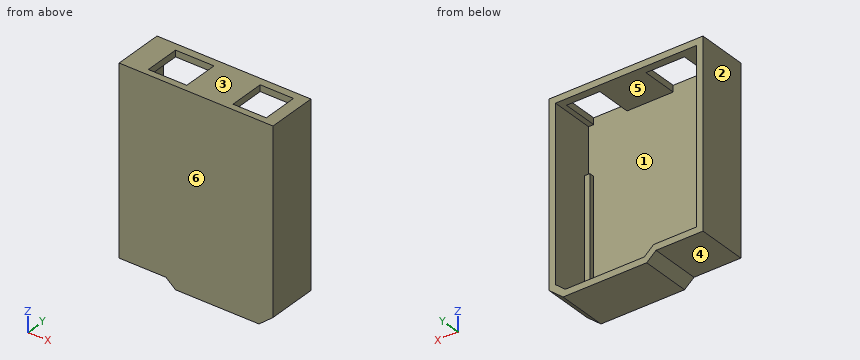
from build123d import *

# Parameters (mm, degrees)
BOSS_EXTRUDE1_DEPTH = 17
SHELL1_T            = 2.5
SKETCH2_W           = 15
SKETCH2_H           = 14
SKETCH2_W_2         = 13
CUT_EXTRUDE1_DEPTH  = 4
SKETCH3_W           = 2
SKETCH3_H           = 50
BOSS_EXTRUDE2_DEPTH = 2
SKETCH4_W           = 26.147040262
SKETCH4_H           = 2.874772828
BOSS_EXTRUDE3_DEPTH = 2


with BuildPart() as part:
    # Sketch1 → Boss-Extrude1 (new body)
    with BuildSketch(Plane(origin=(0, 0, 0), x_dir=(1, 0, 0), z_dir=(0, 1, 0))):
        Polygon((0, 0), (0, 67), (16.729272308, 67), (20.392796314, 70.176839536), (51.157808577, 70.176839536), (55, 67), (55, 0), align=None)
    extrude(amount=BOSS_EXTRUDE1_DEPTH)

    # Shell1
    shell1_openings = [part.faces().sort_by_distance(p)[0] for p in [
        (27.740476626, 17, -34.512318995),
    ]]
    offset(amount=SHELL1_T, openings=shell1_openings, kind=Kind.INTERSECTION)

    # Sketch2 → Cut-Extrude1 (cut)
    with BuildSketch(Plane(origin=(0, 0, 0), x_dir=(-1, 0, 0), z_dir=(0, 0, -1))):
        with Locations((-14.5, 7)):
            Rectangle(SKETCH2_W, SKETCH2_H)
        with Locations((-46.5, 7)):
            Rectangle(SKETCH2_W_2, SKETCH2_H)
    extrude(amount=-CUT_EXTRUDE1_DEPTH, mode=Mode.SUBTRACT)

    # Sketch3 → Boss-Extrude2 (add)
    with BuildSketch(Plane(origin=(0, 0, 0), x_dir=(1, 0, 0), z_dir=(0, 1, 0))):
        with Locations((1, 44.078139118)):
            Rectangle(SKETCH3_W, SKETCH3_H)
        with Locations((54, 44.078139118)):
            Rectangle(SKETCH3_W, SKETCH3_H)
    extrude(amount=BOSS_EXTRUDE2_DEPTH)

    # Sketch4 → Boss-Extrude3 (add)
    with BuildSketch(Plane(origin=(0, 0, 0), x_dir=(1, 0, 0), z_dir=(0, 1, 0))):
        with Locations((35.808300775, 68.739453122)):
            Rectangle(SKETCH4_W, SKETCH4_H)
    extrude(amount=BOSS_EXTRUDE3_DEPTH)


solid = part.part
Source: CAD feature listing. Evaluate the final solid. Frame: model axes, mm. Face numbers are marked on the shaded views. A direction names the side the tool comes from. Give positions to 0.01 mm unless a question says otherwise; leave off trailing zeros. Order: outer loops, then holes, each group sorted by start corner. A loop starts at its lowest first (then second) coordinate and runs counter-clockwise, first axis right, second up. Notation, with made-up numbers: (18.5, -33) -> (30.5, -33) arc R9 ccw to (30.5, -23) -> close; hole circle Ø8 at (-12.5, 62). An arc over 180 degrees is marked (long way). Use a Markdown table: item, result.
1) Contact query for flat-ended pins moving along their axis: P1, Ø1, axis at x = 4.5, z = -42.5, coming from the +Y side; P2, Ø1.6, axis at x = 53.5, z = -55.5, coming from the +Y side; P3, Ø8.5, axis at x = 11.5, y = 9.5, coming from the +Z side. Output: stop coordinate, or through.
Answer list:
| item | result |
|---|---|
| P1 | y = 0 |
| P2 | y = 2 |
| P3 | z = -67 |
2) Section query D-D, the plane x = 29. Return the cut outline in (y, z).
Answer list:
| item | result |
|---|---|
| outline | (-2.5, -72.68) -> (17, -72.68) -> (17, -70.18) -> (2, -70.18) -> (2, -67.3) -> (0, -67.3) -> (0, 0) -> (17, 0) -> (17, 2.5) -> (-2.5, 2.5) -> close |
3) Ray query, line 1 along Z through (x, y) = (28, 2.5); line 2 along X through (y, z) = (15.25, -38); line 3 along Z through (x, y) = (33, 0.5). Return the intervals inside material, ascending. Write a range as [from, to].
Answer list:
| item | result |
|---|---|
| line 1 | [-72.68, -70.18], [0, 2.5] |
| line 2 | [-2.5, 0], [55, 57.5] |
| line 3 | [-72.68, -67.3], [0, 2.5] |
4) Section query B-B, the plane y = 5.75. Return the cut outline in (x, z), then the cut area to 3 significant figures.
Answer list:
| item | result |
|---|---|
| outline | (-2.5, -69.5) -> (15.8, -69.5) -> (19.46, -72.68) -> (52.06, -72.68) -> (57.5, -68.18) -> (57.5, 2.5) -> (53, 2.5) -> (53, 0) -> (55, 0) -> (55, -67) -> (51.16, -70.18) -> (20.39, -70.18) -> (16.73, -67) -> (0, -67) -> (0, 0) -> (7, 0) -> (7, 2.5) -> (-2.5, 2.5) -> close; (22, 0) -> (40, 0) -> (40, 2.5) -> (22, 2.5) -> close |
| area | 570 mm² |
5) Reachability of the marked faces 4, 5 and 6 from +Z, -Z, +X, -X, +Y, -Y: full face, straight path, thin tool, end or side. Return the list, or none.
Answer list:
| item | result |
|---|---|
| face 4 | -Z, -X, +Y, -Y |
| face 5 | +Y |
| face 6 | +Z, -Z, +X, -X, -Y |
6) Section query C-C, the plane z = -64. Return the cut outline in (x, y), then the cut area to 3 significant figures.
Answer list:
| item | result |
|---|---|
| outline | (-2.5, -2.5) -> (57.5, -2.5) -> (57.5, 17) -> (55, 17) -> (55, 2) -> (53, 2) -> (53, 0) -> (2, 0) -> (2, 2) -> (0, 2) -> (0, 17) -> (-2.5, 17) -> close |
| area | 243 mm² |
7) Mould query, pull axis Z, two halves, no side actions, for the marked faces 1, 2 and 3. Classes: +Z half, -Z half, draft (parallel to the pull), parting line (faces both ways), or undercut.
Answer list:
| item | result |
|---|---|
| face 1 | undercut |
| face 2 | draft |
| face 3 | +Z half |
8) Section query A-A, the plane x = 11. Return the cut outline in (y, z).
Answer list:
| item | result |
|---|---|
| outline | (-2.5, -69.5) -> (17, -69.5) -> (17, -67) -> (0, -67) -> (0, 2.5) -> (-2.5, 2.5) -> close; (14, 0) -> (17, 0) -> (17, 2.5) -> (14, 2.5) -> close |
